Could you check a few things on this model? Use its own coordinates, in mm. Face numbers are marked on the shaded views. A direction names the side the tool comes from. Round coordinates to 2 decimals unless told otherwise and drop trailing zeros. Loops run counter-clockwise (first coordinate to the right, second up) from the corner with the lowest first, then second, coordinate; pieces in that order, holes last. Notation, with made-up numbers: (39.5, 70) -> (94.5, 70) arc R14 cw to (94.5, 96) -> close; hole circle Ø4 at (-28.5, 56). An arc over 180 degrees is marked (long way). Use CSV: the item, a comma, the result in double quotes. Start each with the question number.
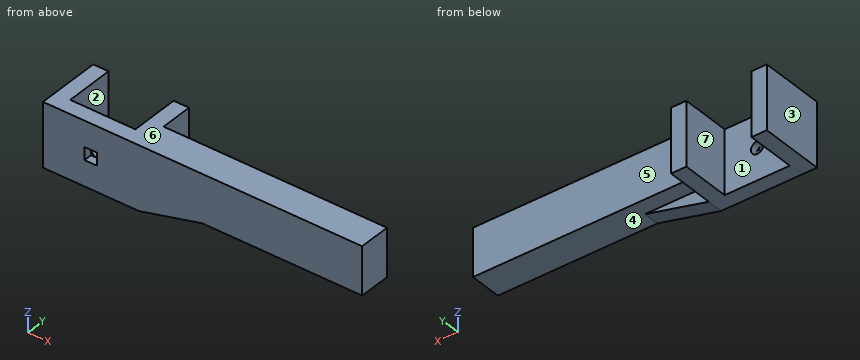
```python
from build123d import *

# Parameters (mm, degrees)
F1_DEPTH = 12.7
F2_R     = 2.5
F3_DEPTH = 25.655
F4_W     = 5.0546
F4_H     = 5.0546
F5_DEPTH = 3.302
F6_W     = 88.9
F6_H     = 12.7
F7_DEPTH = 19.05
F9_DEPTH = 6.35


with BuildPart() as f1:
    # F0 (on Top) → F1 (new body, symmetric)
    with BuildSketch(Plane.XY):
        Polygon((12.954, 9.779), (12.954, -9.779), (-12.954, -9.779), (-12.954, 9.779), (-19.05, 9.779), (-19.05, -15.875), (19.05, -15.875), (19.05, 9.779), align=None)
    extrude(amount=F1_DEPTH, both=True)

    # F2 (on face) → F3 (cut, through all)
    with BuildSketch(Plane.XZ.offset(15.875)):
        Circle(F2_R)
    extrude(amount=-F3_DEPTH, mode=Mode.SUBTRACT)

    # F4 (on face) → F5 (cut)
    with BuildSketch(Plane.XZ.offset(15.875)):
        Rectangle(F4_W, F4_H)
    extrude(amount=-F5_DEPTH, mode=Mode.SUBTRACT)

    # F6 (on face) → F7 (join)
    with BuildSketch(Plane.XY.offset(12.7)):
        with Locations((63.5, -9.525)):
            Rectangle(F6_W, F6_H)
    extrude(amount=-F7_DEPTH)

    # F8 (on face) → F9 (join)
    with BuildSketch(Plane.XZ.offset(15.875)):
        Polygon((19.05, -6.35), (19.05, -12.7), (44.45, -6.35), align=None)
    extrude(amount=-F9_DEPTH)


solid = f1.part
```
1. Will these pins go through, and if not, where does the flat tip stop? pin 1 (3 mm diameter, centred on x = 54.5, z = 2.5, fed in from +Y) (3 decimals); pin 2 (14 mm diameter, centred on x = 63.5, y = -9.5, fed in from -Z); pin 3 (3 mm diameter, centred on x = 33, z = -10.5, fed in from +Y) (3 decimals); pin 4 (2.5 mm diameter, centred on x = 0.5, z = 1, fed in from -Y).
2. If I drill on L1, parallel to X at y = 2.5, z = -7.5; L2, parallel to X at y = -3.5, z = 6; L3, parallel to Z at x = 0, y = -10.6, over which ranges is the centre line in solid material (lowest first)?
3. For the marked faces 5, 6 and 7, which set-ups out of +Z, -Z, +X, -X, +Y, -Y let a thin tool reach every point of the face, with its end or its side?
4. Suppose I cut it at B-B (z = 0). List the corners of the cut face in (x, y) for me (3 decimals).
5. Suppose I cut it at D-D (y = -11.5). List the corners of the cut face in (x, z) for me, then the cut area to 3 significant figures.
6. Suppose I cut it at A-A (y = 2.25). List the corners of the cut face in (x, z) for me.
7. Suppose I cut it at C-C (x = 0). List the corners of the cut face in (y, z) for me (3 decimals).
8. We'd pull the mould along X, two halves only. Please class the marked faces 1, 2, 3 and 4: pulls with the +X half, pulls with the -X half, needs draft (parallel to the pull), parting line crosses it, or undercut.
Geometry check:
1,pin 1,"stops at y = -3.175"
1,pin 2,"stops at z = -6.35"
1,pin 3,"stops at y = -9.525"
1,pin 4,"passes through"
2,L1,"x = -19.05 to -12.95, 12.95 to 19.05"
2,L2,"x = -19.05 to -12.95, 12.95 to 107.95"
2,L3,"z = -12.7 to -2.5, 2.5 to 12.7"
3,face 5,"+Z, -Z, +X, +Y"
3,face 6,"+Z, +X, -X, +Y, -Y"
3,face 7,"+Z, -Z, +Y"
4,outline,"(-19.05, -15.875) -> (-2.527, -15.875) -> (-2.527, -12.573) -> (-2.5, -12.573) -> (-2.5, -9.779) -> (-12.954, -9.779) -> (-12.954, 9.779) -> (-19.05, 9.779) -> close; (2.5, -12.573) -> (2.527, -12.573) -> (2.527, -15.875) -> (107.95, -15.875) -> (107.95, -3.175) -> (19.05, -3.175) -> (19.05, 9.779) -> (12.954, 9.779) -> (12.954, -9.779) -> (2.5, -9.779) -> close"
5,outline,"(-19.05, -12.7) -> (19.05, -12.7) -> (44.45, -6.35) -> (107.95, -6.35) -> (107.95, 12.7) -> (-19.05, 12.7) -> close; hole circle Ø5 at (0, 0)"
5,area,"2,720 mm²"
6,outline,"(-19.05, -12.7) -> (-12.95, -12.7) -> (-12.95, 12.7) -> (-19.05, 12.7) -> close; (12.95, -12.7) -> (19.05, -12.7) -> (19.05, 12.7) -> (12.95, 12.7) -> close"
7,outline,"(-15.875, -12.7) -> (-9.779, -12.7) -> (-9.779, -2.5) -> (-12.573, -2.5) -> (-12.573, -2.527) -> (-15.875, -2.527) -> close; (-15.875, 2.527) -> (-12.573, 2.527) -> (-12.573, 2.5) -> (-9.779, 2.5) -> (-9.779, 12.7) -> (-15.875, 12.7) -> close"
8,face 1,"undercut"
8,face 2,"undercut"
8,face 3,"pulls with the -X half"
8,face 4,"needs draft"
